CAD build for the part. Positions are in the model's coordinates, mm. Face numbers are marked on the shaded views. A direction names the side the tool comes from. Round coordinates to 2 decimals unless told otherwise and drop trailing zeros. Order: outer loops, then holes, each group sorted by start corner. A loop starts at its lowest first (then second) coordinate and runs counter-clockwise, first axis right, second up.
```python
from build123d import *

# Parameters (mm, degrees)
SKETCH1_W           = 31.26
SKETCH1_H           = 32.08
BOSS_EXTRUDE2_DEPTH = 1.61
SKETCH4_W           = 31.26
SKETCH4_H           = 32.08
SKETCH4_W_2         = 27.26
SKETCH4_H_2         = 28.08
BOSS_EXTRUDE3_DEPTH = 5
SKETCH5_W           = 14
SKETCH5_H           = 5
CUT_EXTRUDE3_DEPTH  = 5
SKETCH8_W           = 14
SKETCH8_H           = 3
CUT_EXTRUDE5_DEPTH  = 5
SKETCH9_W           = 31.26
SKETCH9_H           = 32.08
BOSS_EXTRUDE4_DEPTH = 3
SKETCH10_R          = 2.5
CUT_EXTRUDE6_DEPTH  = 2


with BuildPart() as part:
    # Sketch1 → Boss-Extrude2 (new body)
    with BuildSketch(Plane(origin=(0, 0, 0), x_dir=(1, 0, 0), z_dir=(0, 1, 0))):
        with Locations((2.801725352, -6.324753521)):
            Rectangle(SKETCH1_W, SKETCH1_H)
    extrude(amount=BOSS_EXTRUDE2_DEPTH)

    # Sketch4 → Boss-Extrude3 (add)
    with BuildSketch(Plane(origin=(0, 1.61, 0), x_dir=(1, 0, 0), z_dir=(0, 1, 0))):
        with Locations((2.801725352, -6.324753521)):
            Rectangle(SKETCH4_W, SKETCH4_H)
        with Locations((2.801725352, -6.324753521)):
            Rectangle(SKETCH4_W_2, SKETCH4_H_2, mode=Mode.SUBTRACT)
    extrude(amount=BOSS_EXTRUDE3_DEPTH)

    # Sketch5 → Cut-Extrude3 (cut)
    with BuildSketch(Plane(origin=(0, 1.61, 0), x_dir=(1, 0, 0), z_dir=(0, 1, 0))):
        with Locations((2.801725352, 5.215246479)):
            Rectangle(SKETCH5_W, SKETCH5_H)
    extrude(amount=-CUT_EXTRUDE3_DEPTH, mode=Mode.SUBTRACT)

    # Sketch8 → Cut-Extrude5 (cut)
    with BuildSketch(Plane(origin=(0, 0, -9.715246479), x_dir=(-1, 0, 0), z_dir=(0, 0, -1))):
        with Locations((-2.801725352, 1.5)):
            Rectangle(SKETCH8_W, SKETCH8_H)
    extrude(amount=-CUT_EXTRUDE5_DEPTH, mode=Mode.SUBTRACT)

    # Sketch9 → Boss-Extrude4 (add)
    with BuildSketch(Plane.XZ):
        with Locations((2.801725352, 6.324753521)):
            Rectangle(SKETCH9_W, SKETCH9_H)
    extrude(amount=BOSS_EXTRUDE4_DEPTH)

    # Sketch10 → Cut-Extrude6 (cut)
    with BuildSketch(Plane.XZ.offset(3)):
        with Locations((2.801725352, 15.644753521)):
            Circle(SKETCH10_R)
        with Locations((11.101725352, 6.324753521)):
            Circle(SKETCH10_R)
        with Locations((-5.498274648, 6.324753521)):
            Circle(SKETCH10_R)
        with Locations((2.801725352, -2.995246479)):
            Circle(SKETCH10_R)
    extrude(amount=-CUT_EXTRUDE6_DEPTH, mode=Mode.SUBTRACT)


solid = part.part
```
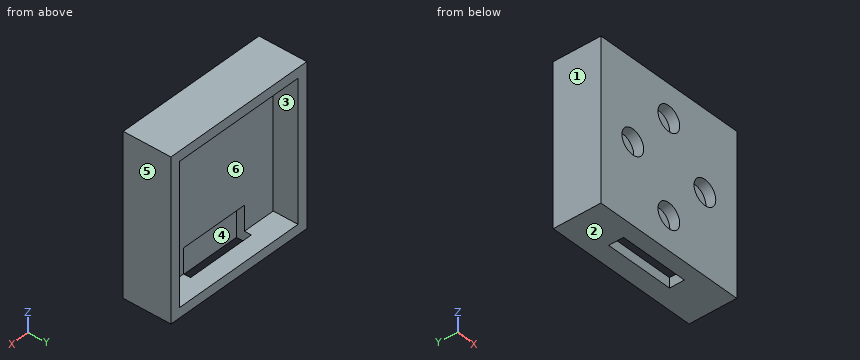
1. Cut at A-A, the plane x = -2.5. Write the cut outline in (y, z), and give its area (3 significant figures).
2. Drill centre lines: line 1 (X direction, y = 1.5, z = -5); line 2 (Y direction, x = 7.5, z = -8); line 3 (Z direction, x = 1, y = 6). Where is each one in solid material? Low to high.
3. Tool access for the marked faces 4, 5 and 6: list every direction of +Z, -Z, +X, -X, +Y, -Y with a clear straight run to the whole face (end or side of a thin tool).
4. Cut at D-D, the plane z = -1. Write the cut outline in (x, y).
5. Cut at C-C, the plane y = 2.25. Write the cut outline in (x, z), and give its area (3 significant figures).
6. Pin check, flat tips, straight feed: P1, Ø3, axis at x = 2.8, z = -3, coming from the +Y side; P2, Ø1.5, axis at x = -4.5, z = 5, coming from the -Y side. Stop position of each tip, or through.
7. Mould opens along Z. For the marked faces 1, 2 and 3 say: released by +Z, released by -Z, zero draft, split by the parting line, or undercut.
8. Cut at B-B, the plane y = 5.5. Write the cut outline in (x, z), and give its area (3 significant figures).
Outcome:
1. outline: (-3, -9.72) - (0, -9.72) - (0, -2.72) - (1.61, -2.72) - (1.61, 20.36) - (6.61, 20.36) - (6.61, 22.36) - (-3, 22.36) - close; (3, -9.72) - (6.61, -9.72) - (6.61, -7.72) - (3, -7.72) - close
1. area: 154 mm2
2. line 1: x = -12.83 to -4.2, 9.8 to 18.43
2. line 2: y = -3 to 0, 3 to 6.61
2. line 3: z = -9.72 to -7.72, 20.36 to 22.36
3. face 4: -Z
3. face 5: +Z, -Z, +X, +Y, -Y
3. face 6: +Y
4. outline: (-12.83, -3) - (1.3, -3) - (1.3, -1) - (4.31, -1) - (4.31, -3) - (18.43, -3) - (18.43, 6.61) - (16.43, 6.61) - (16.43, 1.61) - (-10.83, 1.61) - (-10.83, 6.61) - (-12.83, 6.61) - close
5. outline: (-12.83, -9.72) - (-4.2, -9.72) - (-4.2, -7.72) - (-10.83, -7.72) - (-10.83, 20.36) - (16.43, 20.36) - (16.43, -7.72) - (9.8, -7.72) - (9.8, -9.72) - (18.43, -9.72) - (18.43, 22.36) - (-12.83, 22.36) - close
5. area: 209 mm2
6. P1: stops at y = 1.61
6. P2: stops at y = -1
7. face 1: zero draft
7. face 2: released by -Z
7. face 3: undercut
8. outline: (-12.83, -9.72) - (18.43, -9.72) - (18.43, 22.36) - (-12.83, 22.36) - close; hole (-10.83, -7.72) - (16.43, -7.72) - (16.43, 20.36) - (-10.83, 20.36) - close
8. area: 237 mm2
